Design review of the part built by this model. Coordinates are the model's own, in mm. Face numbers are marked on the shaded views. A direction names the side the tool comes from. Round coordinates to 2 decimals unless told otherwise and drop trailing zeros. Loops run counter-clockwise (first coordinate to the right, second up) from the corner with the lowest first, then second, coordinate; pieces in that order, holes last. Notation, with made-up numbers: M 78,16 L 108,16 A22 ccw 108,29 Z; hole C 10,27.25 d11. An arc over 180 degrees is marked long. Use a Markdown table: item, result.
Autodesk Inventor part; units mm, degrees
ref_plane "YZ Plane" through (0, 0, 0) normal (1, 0, 0) x (0, 1, 0)
ref_plane "XZ Plane" through (0, 0, 0) normal (0, 1, 0) x (-1, 0, 0)
ref_plane "XY Plane" through (0, 0, 0) normal (0, 0, 1) x (1, 0, 0)
sketch "スケッチ1" plane through (0, 0, 0) normal (0, 1, 0) x (-1, 0, 0)
  line L0 (75, 0) -> (105, -51.9615)
  line L1 (-75, 0) -> (-105, -51.9615)
  line L2 (0, -218.2384) -> (0, 36.3731)
  line L3 (147, 0) -> (-147, 0)
  line L4 (105, -51.9615) -> (30, -181.8653)
  line L5 (30, -181.8653) -> (-30, -181.8653)
  line L6 (-30, -181.8653) -> (-105, -51.9615)
  line L7 (75, 0) -> (-75, 0)
  line L8 (34, 0) -> (34, -24.3509)
  line L9 (34, -24.3509) -> (48.7058, -49.822)
  line L10 (48.7058, -49.822) -> (90, -25.9808)
  line L11 (45, 0) -> (45, -18) construction
  line L12 (45, -18) -> (34, -24.3509) construction
  line L13 (84.5, -87.4686) -> (63.4115, -75.2931)
  line L14 (63.4115, -75.2931) -> (48.7058, -49.822)
  line L15 (-34, 0) -> (-34, -24.3509)
  line L16 (-34, -24.3509) -> (-48.7058, -49.822)
  line L17 (-63.4115, -75.2931) -> (-48.7058, -49.822)
  line L18 (-84.5, -87.4686) -> (-63.4115, -75.2931)
  circle A0 centre (30, -32.75) radius 1.6
  circle A1 centre (-30, -32.75) radius 1.6
  line L19 (35.5295, -27) -> (-35.5295, -27)
  point P0 (0, 0)
  point P1 (0, 0)
  point P2 (0, -27)
  dimension "d1" = 150
  dimension "d2" = 60
  dimension "d3" = 60
  dimension "d6" = 60
  dimension "d30" = 60
  dimension "d31" = 18
  dimension "d32" = 30
  dimension "d33" = 41
  dimension "d34" = 3.2
  dimension "d35" = 30
  dimension "d36" = 32.75
  dimension "d37" = 27
extrude "プレート1" add sketch "スケッチ1" along normal blind 1.5 contours L14 L13 L4 L5 L2 L19 L9 | L2 L5 L6 L18 L17 L16 L19
sketch "スケッチ4" plane through (0, 1.5, 0) normal (0, 1, 0) x (1, 0, 0)
  circle A0 centre (30, 67.8013) radius 1.6
  circle A1 centre (45, 67.8013) radius 1.6
  line L0 (0, 218.2384) -> (0, -36.3731)
  circle A2 centre (-30, 67.8013) radius 1.6
  circle A3 centre (-45, 67.8013) radius 1.6
  line L1 (61.6173, 73.1025) -> (25, 73.1025)
  line L2 (25, 73.1025) -> (25, 62.5)
  line L3 (-61.6173, 73.1025) -> (-25, 73.1025)
  line L4 (-25, 73.1025) -> (-25, 62.5)
  line L5 (-25, 62.5) -> (25, 62.5)
  line L6 (-30, 73.1025) -> (30, 73.1025)
  line L7 (30, 73.1025) -> (30, 181.8653)
  line L8 (30, 181.8653) -> (-30, 181.8653)
  line L9 (-30, 181.8653) -> (-30, 73.1025)
  line L10 (-25, 62.5) -> (25, 62.5)
  line L11 (25, 62.5) -> (25, 73.1025)
  line L12 (25, 73.1025) -> (-25, 73.1025)
  line L13 (-25, 73.1025) -> (-25, 62.5)
  line L14 (30, 181.8653) -> (84.5, 87.4686)
  line L15 (70, 112.5833) -> (30, 89.4893)
  line L16 (-30, 89.4893) -> (-70, 112.5833)
  line L17 (-84.5, 87.4686) -> (-30, 181.8653)
  line L18 (84.5, 87.4686) -> (63.4115, 75.2931)
  line L19 (-63.4115, 75.2931) -> (-84.5, 87.4686)
  line L20 (-35.5295, 27) -> (-63.4115, 75.2931)
  point P0 (0, 0)
  dimension "d40" = 80
extrude "切り取り3" cut sketch "スケッチ4" against normal blind 1.5
sketch "スケッチ5" plane through (0, 1.5, 0) normal (0, 1, 0) x (1, 0, 0)
  line L0 (-75, 44) -> (75, 44)
  circle A0 centre (-20, 41) radius 3
  circle A1 centre (20, 41) radius 3
  line L1 (-25, 62.5) -> (25, 62.5)
  line L2 (0, 62.5) -> (0, 27)
  line L3 (35.5295, 27) -> (-35.5295, 27)
  circle A2 centre (-20, 41) radius 1.6
  circle A3 centre (20, 41) radius 1.6
  circle A4 centre (0, 34) radius 1.6
  point P0 (0, 0)
  dimension "d41" = 6
  dimension "d42" = 6
  dimension "d43" = 40
  dimension "d44" = 3.2
  dimension "d45" = 3.2
  dimension "d46" = 3.2
  dimension "d47" = 7
extrude "切り取り4" cut sketch "スケッチ5" against normal blind 1.5 contours A4 L2 | L2 A4 | A2 | A3
sketch "スケッチ6" plane through (0, 1.5, 0) normal (0, 1, 0) x (1, 0, 0)
  circle A0 centre (-20, 41) radius 1.6
  circle A1 centre (20, 41) radius 1.6
  circle A2 centre (-20, 41) radius 3
  circle A3 centre (20, 41) radius 3
  line L0 (-70.724, 59) -> (85.6586, 59)
  line L1 (85.6586, 59) -> (85.6586, 44)
  line L2 (85.6586, 44) -> (-70.724, 44)
  line L3 (-70.724, 44) -> (-70.724, 59)
  circle A4 centre (0, 34) radius 1.6
  circle A5 centre (0, 34) radius 10
  circle A6 centre (-20, 41) radius 6
  circle A7 centre (20, 41) radius 6
  line L4 (-5.0258, 25.3547) -> (-23.0155, 35.8128)
  line L5 (5.0258, 25.3547) -> (23.0155, 35.8128)
  line L6 (35.5295, 27) -> (-35.5295, 27)
  line L7 (-25, 27) -> (-25, 44)
  line L8 (25, 27) -> (25, 44)
  circle A8 centre (-30, 32.75) radius 1.6
  circle A9 centre (30, 32.75) radius 1.6
  line L9 (-25, 73.1025) -> (-25, 62.5)
  line L10 (-25, 62.5) -> (-25, 59)
  line L11 (-25, 62.5) -> (25, 62.5)
  line L12 (25, 62.5) -> (25, 59)
  point P0 (0, 0)
  point P1 (25, 37.6834)
  point P2 (7.856, 27)
  point P3 (-25, 37.6834)
  point P4 (-7.856, 27)
  dimension "d52" = 12
  dimension "d53" = 12
  dimension "d50" = 6
  dimension "d51" = 15
  dimension "d54" = 5
  dimension "d55" = 5
extrude "押し出し1" add sketch "スケッチ6" along normal blind 11.8 contours A6 L4 L6 L7 | A7 L8 L6 L5 | L10 L11 L12 L0
sketch "スケッチ7" plane through (0, 1.5, 0) normal (0, 1, 0) x (1, 0, 0)
  line L0 (-176.5784, 180.8905) -> (313.8631, 180.8905)
  line L1 (313.8631, 180.8905) -> (313.8631, -72.7571)
  line L2 (313.8631, -72.7571) -> (-176.5784, -72.7571)
  line L3 (-176.5784, -72.7571) -> (-176.5784, 180.8905)
  point P0 (0, 0)
extrude "押し出し2" cut sketch "スケッチ7" against normal through all
sketch "スケッチ8" plane through (25, 13.3, -62.5) normal (0, 0, -1) x (-1, 0, 0)
  line L0 (0, -11.8) -> (50, -11.8)
  line L1 (0, -11.8) -> (50, -11.8)
  line L2 (50, -11.8) -> (50, 2.7)
  line L3 (50, 2.7) -> (0, 2.7)
  line L4 (0, 2.7) -> (0, -11.8)
  line L5 (50, -11.8) -> (50, 0)
  line L6 (0, 0) -> (50, 0)
  point P0 (25, -13.3)
  dimension "d60" = 2.7
extrude "押し出し3" add sketch "スケッチ8" along normal blind 1.5
sketch "スケッチ9" plane through (25, 13.3, -62.5) normal (0, 0, 1) x (1, 0, 0)
  line L0 (-50, 0) -> (-50, 2.7)
  line L1 (-50, 2.7) -> (0, 2.7)
  line L2 (0, 2.7) -> (0, 1.7)
  line L3 (0, 1.7) -> (-50, 1.7)
  line L4 (-50, 1.7) -> (-50, 2.7)
  line L5 (0, 2.7) -> (0, 0)
  point P0 (-25, -13.3)
  dimension "d63" = 1
extrude "押し出し4" add sketch "スケッチ9" along normal blind 2
sketch "スケッチ11" plane through (0, 13.3, 0) normal (0, 1, 0) x (1, 0, 0)
  line L0 (-7.856, 27) -> (-23.0155, 35.8128)
  line L1 (23.0155, 35.8128) -> (7.856, 27)
  circle A0 centre (0, 34) radius 10
  circle A1 centre (0, 34) radius 13
  line L2 (-7.856, 27) -> (-5.0258, 25.3547)
  line L3 (7.856, 27) -> (5.0258, 25.3547)
  point P0 (0, 0)
  point P1 (-12.2072, 29.5295)
  point P2 (12.2072, 29.5295)
  dimension "d66" = 20
  dimension "d67" = 26
extrude "押し出し5" add sketch "スケッチ11" against normal blind 3 contours L2 A0 L3 L1 A1 L0 picked at (-6.6023, 24.0668)
sketch "スケッチ12" plane through (0, 13.3, 0) normal (0, 1, 0) x (1, 0, 0)
  circle A0 centre (-22, 30) radius 1.6
  circle A1 centre (22, 30) radius 1.6
  line L0 (25, 60.5) -> (-25, 60.5)
  line L1 (0, 60.5) -> (0, 48.3991)
  line L2 (-25, 27) -> (-10.9545, 27)
  line L3 (-25, 37.6834) -> (-25, 27)
  point P0 (0, 0)
  dimension "d70" = 3.2
  dimension "d71" = 3
  dimension "d72" = 3
extrude "押し出し6" cut sketch "スケッチ12" against normal through all
sketch "スケッチ13" plane through (0, 1.5, 0) normal (0, -1, 0) x (1, 0, 0)
  line L0 (-25, -37.6834) -> (-25, -27)
  line L1 (-25, -27) -> (25, -27)
  line L2 (25, -27) -> (25, -64)
  line L3 (25, -64) -> (-25, -64)
  line L4 (-25, -64) -> (-25, -27)
  circle A0 centre (-22, -30) radius 1.6
  circle A1 centre (22, -30) radius 1.6
  point P0 (0, 0)
extrude "押し出し7" add sketch "スケッチ13" along normal blind 2
sketch "スケッチ14" plane through (0, -0.5, 0) normal (0, -1, 0) x (1, 0, 0)
  circle A0 centre (-20, -41) radius 1.6
  circle A1 centre (0, -34) radius 1.6
  circle A2 centre (20, -41) radius 1.6
  line L0 (-30, -73.9008) -> (-76.75, -100.892)
  line L1 (-84.5, -87.4686) -> (-76.75, -100.892)
  line L2 (-63.4115, -75.2931) -> (-84.5, -87.4686)
  line L3 (-35.5295, -27) -> (-63.4115, -75.2931)
  line L4 (35.5295, -27) -> (-35.5295, -27)
  line L5 (63.4115, -75.2931) -> (35.5295, -27)
  line L6 (84.5, -87.4686) -> (63.4115, -75.2931)
  line L7 (76.75, -100.892) -> (84.5, -87.4686)
  line L8 (76.75, -100.892) -> (30, -73.9008)
  line L9 (30, -73.9008) -> (30, -73.1025)
  line L10 (30, -73.1025) -> (25, -73.1025)
  line L11 (25, -73.1025) -> (25, -62.5)
  line L12 (25, -62.5) -> (-25, -62.5)
  line L13 (-25, -62.5) -> (-25, -73.1025)
  line L14 (-25, -73.1025) -> (-30, -73.1025)
  line L15 (-30, -73.1025) -> (-30, -73.9008)
  circle A3 centre (-30, -67.8013) radius 1.6
  circle A4 centre (30, -67.8013) radius 1.6
  circle A5 centre (45, -67.8013) radius 1.6
  circle A6 centre (-45, -67.8013) radius 1.6
  circle A7 centre (30, -32.75) radius 1.6
  circle A8 centre (-30, -32.75) radius 1.6
  circle A9 centre (48.4391, -79.9279) radius 1.6
  circle A10 centre (-48.4391, -79.9279) radius 1.6
  circle A11 centre (-73.3666, -93.1522) radius 1.6
  circle A12 centre (73.3666, -93.1522) radius 1.6
  point P0 (0, 0)
extrude "押し出し8" cut sketch "スケッチ14" against normal through all contours A0 | A1 | A2
sketch "スケッチ15" plane through (0, -0.5, 0) normal (0, -1, 0) x (1, 0, 0)
  line L0 (3.2909, -34) -> (1.6454, -36.85)
  line L1 (1.6454, -36.85) -> (-1.6454, -36.85)
  line L2 (-1.6454, -36.85) -> (-3.2909, -34)
  line L3 (-3.2909, -34) -> (-1.6454, -31.15)
  line L4 (-1.6454, -31.15) -> (1.6454, -31.15)
  line L5 (1.6454, -31.15) -> (3.2909, -34)
  line L6 (21.6454, -43.85) -> (18.3546, -43.85)
  line L7 (18.3546, -43.85) -> (16.7091, -41)
  line L8 (16.7091, -41) -> (18.3546, -38.15)
  line L9 (18.3546, -38.15) -> (21.6454, -38.15)
  line L10 (21.6454, -38.15) -> (23.2909, -41)
  line L11 (23.2909, -41) -> (21.6454, -43.85)
  line L12 (-16.7091, -41) -> (-18.3546, -43.85)
  line L13 (-18.3546, -43.85) -> (-21.6454, -43.85)
  line L14 (-21.6454, -43.85) -> (-23.2909, -41)
  line L15 (-23.2909, -41) -> (-21.6454, -38.15)
  line L16 (-21.6454, -38.15) -> (-18.3546, -38.15)
  line L17 (-18.3546, -38.15) -> (-16.7091, -41)
  circle A0 centre (-20, -41) radius 1.6
  circle A1 centre (0, -34) radius 1.6
  circle A2 centre (20, -41) radius 1.6
  circle A3 centre (20, -41) radius 1.6
  circle A4 centre (0, -34) radius 1.6
  circle A5 centre (-20, -41) radius 1.6
  line L18 (25, -64) -> (25, -27)
  line L19 (25, -27) -> (-25, -27)
  line L20 (-25, -27) -> (-25, -64)
  line L21 (-25, -64) -> (25, -64)
  circle A6 centre (-22, -30) radius 1.6
  circle A7 centre (22, -30) radius 1.6
  point P0 (0, 0)
  point P1 (0, -34)
  point P2 (20, -41)
  point P3 (-20, -41)
  dimension "d80" = 5.7
extrude "押し出し9" add sketch "スケッチ15" along normal blind 1 contours L21 L20 L19 L18
equation "\"d3\" = d2"
equation "\"d38\" = Thickness"
equation "\"d41\" = d42"
equation "\"d48\" = Thickness"
equation "\"d16\" = Thickness"
equation "\"BendRadius\" = Thickness"
equation "\"BendReliefWidth\" = Thickness"
equation "\"BendReliefDepth\" = 0.5 * Thickness"
equation "\"CornerReliefSize\" = 4 * Thickness"
equation "\"MinimumRemnant\" = 2 * Thickness"
equation "\"TransitionRadius\" = BendRadius"
equation "\"JacobiRadiusSize\" = BendRadius"
equation "\"GapSize\" = Thickness"
properties part number "belt_cover_middle"
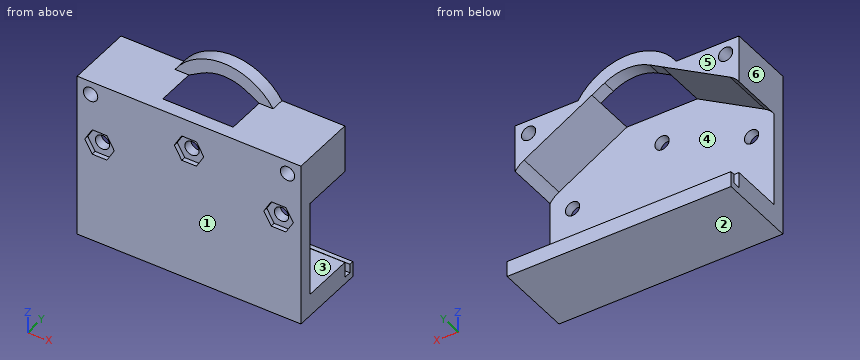
1. Take a section at B-B on z = -42. Give the boundary of the cut face in (x, y).
Check values:
| item | result |
|---|---|
| outline | M -25,-1.5 L -22.71,-1.5 L -22.71,-0.5 L -21.25,-0.5 L -21.25,1.5 L -25,1.5 Z; M -18.75,-0.5 L -17.29,-0.5 L -17.29,-1.5 L 17.29,-1.5 L 17.29,-0.5 L 18.75,-0.5 L 18.75,1.5 L -18.75,1.5 Z; M 21.25,-0.5 L 22.71,-0.5 L 22.71,-1.5 L 25,-1.5 L 25,1.5 L 21.25,1.5 Z |
2. Insertion check: pin 1 (1.1 mm diameter, centred on x = 19.5, y = -1, fed in from +Z); pin 2 (8.5 mm diameter, centred on x = -11, z = -32.5, fed in from +Y); pin 3 (4 mm diameter, centred on x = 6.5, y = 10.5, fed in from +Z). Each pin has a flat end and moves straight along its axis. Give the tip position at first contact, or say it passes through.
Check values:
| item | result |
|---|---|
| pin 1 | stops at z = -27 |
| pin 2 | stops at y = 13.3 |
| pin 3 | stops at z = -21.8 |
3. Machinability: for the marked faces 4, 5 and 6, which of the approach directions +Z, -Z, +X, -X, +Y, -Y give a long, thin tool a straight path to every point of the face, cutting with its end or side? Answer none if there is none.
Check values:
| item | result |
|---|---|
| face 4 | +Y |
| face 5 | +Z, +X, -X, +Y |
| face 6 | +Z, -Z, -X, +Y, -Y |
4. Take a section at C-C on x = -19. Give the boundary of the cut face in (y, z).
Check values:
| item | result |
|---|---|
| outline | M -1.5,-64 L 16,-64 L 16,-60.5 L 15,-60.5 L 15,-62.5 L 13.3,-62.5 L 13.3,-59 L 1.5,-59 L 1.5,-42.25 L -0.5,-42.25 L -0.5,-43.85 L -1.5,-43.85 Z; M -1.5,-38.15 L -0.5,-38.15 L -0.5,-39.75 L 1.5,-39.75 L 1.5,-33.48 L 13.3,-33.48 L 13.3,-27 L -1.5,-27 Z |
5. Wall thickness on line 1 along X through (y, z) = (-1, -30); line 2 along Z through (x, y) = (-20, 0.1); line 3 along X through (y, z) = (8.75, -30): over which ranges is each line inside the solid? List them lowest first. Write a range as from..to.
Check values:
| item | result |
|---|---|
| line 1 | x = -25..-23.6, -20.4..20.4, 23.6..25 |
| line 2 | z = -64..-42.6, -39.4..-27 |
| line 3 | x = -25..-23.6, -20.4..-13.02, 13.02..20.4, 23.6..25 |
6. Take a section at D-D on z = -56. Give the boundary of the cut face in (x, y), and give its area (3 significant figures).
Check values:
| item | result |
|---|---|
| outline | M -25,-1.5 L 25,-1.5 L 25,1.5 L -25,1.5 Z |
| area | 150 mm² |
7. Take a section at A-A on y = 8. Give the boundary of the cut face in (x, z), and give its area (3 significant figures).
Check values:
| item | result |
|---|---|
| outline | M -25,-64 L 25,-64 L 25,-59 L -25,-59 Z; M -25,-37.68 A6 cw -23.02,-35.81 L -7.86,-27 L -25,-27 Z; M 7.86,-27 L 23.02,-35.81 A6 cw 25,-37.68 L 25,-27 Z; hole C -22,-30 d3.2; hole C 22,-30 d3.2 |
| area | 406 mm² |
8. The part is to be moulded in two halves that separate along Z. For the marked faces 1, 2 and 3, say which applies: pulls with the +Z half, pulls with the -Z half, needs draft (parallel to the pull), parting line crosses it, or undercut.
Check values:
| item | result |
|---|---|
| face 1 | needs draft |
| face 2 | pulls with the -Z half |
| face 3 | undercut |
